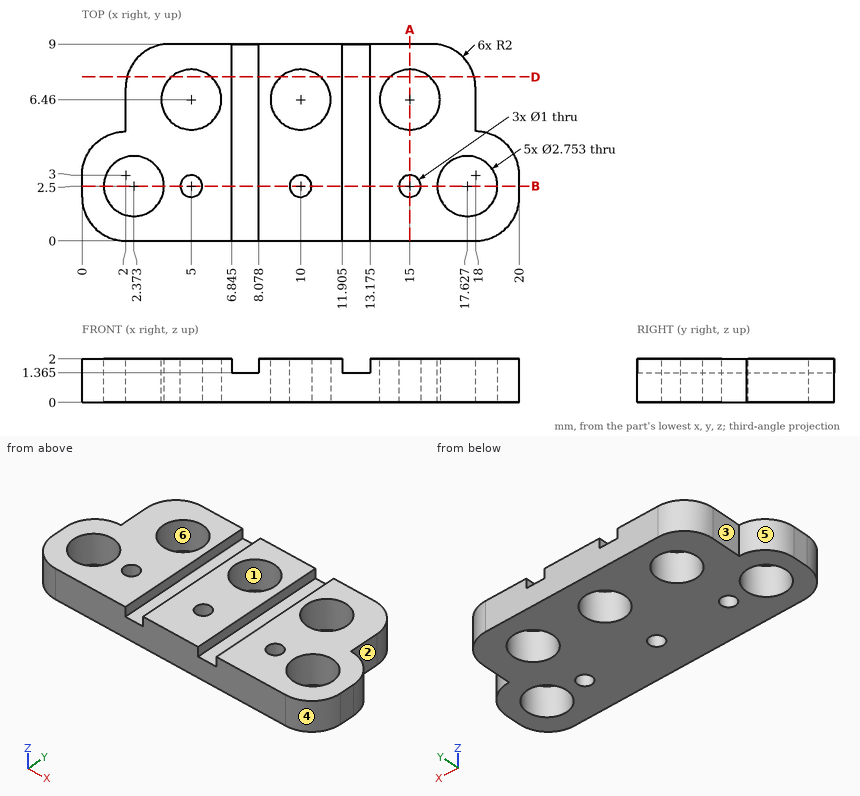
Answer from the drawing. Dimensions are ordinates in mm from the lowest x, y and z of the part. A direction names the side the tool comes from. Give positions to 0.01 mm unless a question says otherwise; leave off trailing zeros. Loops run counter-clockwise (first coordinate to the right, second up) from the corner with the lowest first, then second, coordinate; pieces in that order, holes last.
Item 1: The part is cut by section A-A (x = 15). Write down the section's boundary in (y, z).
Item 2: Find the intervals of material crossed by line 1 along Y through (x, z) = (10, 1.5); line 2 along X through (y, z) = (6.5, 0.1) (1 decimal); line 3 along X through (y, z) = (6.75, 1.5) (1 decimal), in increasing order.
Item 3: The part is cut by section B-B (y = 2.5). Give the number of separate pieces and of enclosed holes in the cut face, and give its area (3 significant figures).
Item 4: Each of these flat-tipped pins is pushed along its axis until it touches: pin 1 Ø0.5 at (y, z) = (5.5, 2) entering from +X; pin 2 Ø1 at (x, y) = (7.5, 4.5) entering from +Z (3 decimals); pin 3 Ø0.6 at (y, z) = (6.5, 1) entering from -X. Where does it stop, or does it pass through?
Item 5: For the marked faces 1, 2 and 3, determine the directions among +Z, -Z, +X, -X, +Y, -Y from which every point of the face is accessible in a straight line to the end or side of a thin tool.
Item 6: The part is cut by section D-D (y = 7.5). Write down the section's boundary in (x, z) (1 decimal).
Item 7: The mould has two halves that part along Y. Classify the marked faces 4, 5 and 6: released by +Y, released by -Y, zero draft, split by the parting line, or undercut.
Taken from the geometry:
1. outline: (0, 0) - (2, 0) - (2, 2) - (0, 2) - close; (3, 0) - (5.08, 0) - (5.08, 2) - (3, 2) - close; (7.84, 0) - (9, 0) - (9, 2) - (7.84, 2) - close
2. line 1: y = 0 to 2, 3 to 5.08, 7.84 to 9
2. line 2: x = 2 to 3.6, 6.4 to 8.6, 11.4 to 13.6, 16.4 to 18
2. line 3: x = 2 to 3.7, 6.3 to 6.8, 8.1 to 8.7, 11.3 to 11.9, 13.2 to 13.7, 16.3 to 18
3. separate pieces: 6
3. enclosed holes: 0
3. area: 21.4 mm2
4. pin 1: stops at x = 18
4. pin 2: stops at z = 1.365
4. pin 3: stops at x = 2
5. face 1: +Z, -Z
5. face 2: +Z, -Z, +X, +Y
5. face 3: +Z, -Z, -X, +Y
6. outline: (2.1, 0) - (4.1, 0) - (4.1, 2) - (2.1, 2) - close; (5.9, 0) - (9.1, 0) - (9.1, 2) - (8.1, 2) - (8.1, 1.4) - (6.8, 1.4) - (6.8, 2) - (5.9, 2) - close; (10.9, 0) - (14.1, 0) - (14.1, 2) - (13.2, 2) - (13.2, 1.4) - (11.9, 1.4) - (11.9, 2) - (10.9, 2) - close; (15.9, 0) - (17.9, 0) - (17.9, 2) - (15.9, 2) - close
7. face 4: released by -Y
7. face 5: released by +Y
7. face 6: undercut
